The listing builds one solid part. Answer for the finished solid, in the listing's coordinates (mm). A direction names the side the tool comes from. Coordinates: 2 decimals unless noted, no trailing zeros. Loops run counter-clockwise (first coordinate to the right, second up) from the corner with the lowest first, then second, coordinate; pieces in that order, holes last. Notation, with made-up numbers: M -15,37 L 36,37 A15 cw 36,49 Z; hole C -29.5,62 d6. An arc over 180 degrees is marked long. Answer in a Markdown table with one row per item. Add a question column.
from build123d import *

# Parameters (mm, degrees)
CYLINDER_R             = 10
CYLINDER_DEPTH         = 10
CYLINDER001_R          = 2
CYLINDER001_DEPTH      = 30
CYLINDER001_ROLL_ANGLE = -90
CYLINDER003_R          = 1.5
CYLINDER003_DEPTH      = 10
CYLINDER003_ROLL_ANGLE = -90
CYLINDER002_R          = 1.5
CYLINDER002_DEPTH      = 10
CYLINDER002_ROLL_ANGLE = -90
BOX001_W               = 15
BOX001_H               = 10
BOX001_DEPTH           = 10
BOX_W                  = 35
BOX_H                  = 30
BOX_DEPTH              = 10
BOX002_W               = 68
BOX002_H               = 10
BOX002_DEPTH           = 10


with BuildPart() as cylinder:
    # Cylinder → Cylinder (new body)
    with BuildSketch(Plane.XY.offset(-5)):
        Circle(CYLINDER_R)
    extrude(amount=CYLINDER_DEPTH)


with BuildPart() as cylinder001:
    # Cylinder001 → Cylinder001 (new body)
    with BuildSketch(Plane.XY):
        Circle(CYLINDER001_R)
    extrude(amount=CYLINDER001_DEPTH)


with BuildPart() as cylinder001_1:
    # Cylinder001 roll: moved
    add(cylinder001.part.rotate(Axis((0, 0, 0), (1, 0, 0)), CYLINDER001_ROLL_ANGLE))


with BuildPart() as cylinder001_2:
    # Cylinder001 placement: moved
    add(cylinder001_1.part.moved(Location((-15, -15, 0))))


with BuildPart() as cylinder003:
    # Cylinder003 → Cylinder003 (new body)
    with BuildSketch(Plane.XY):
        Circle(CYLINDER003_R)
    extrude(amount=CYLINDER003_DEPTH)


with BuildPart() as cylinder003_1:
    # Cylinder003 roll: moved
    add(cylinder003.part.rotate(Axis((0, 0, 0), (1, 0, 0)), CYLINDER003_ROLL_ANGLE))


with BuildPart() as cylinder003_2:
    # Cylinder003 placement: moved
    add(cylinder003_1.part.moved(Location((52, 10, 0))))


with BuildPart() as cylinder002:
    # Cylinder002 → Cylinder002 (new body)
    with BuildSketch(Plane.XY):
        Circle(CYLINDER002_R)
    extrude(amount=CYLINDER002_DEPTH)


with BuildPart() as cylinder002_1:
    # Cylinder002 roll: moved
    add(cylinder002.part.rotate(Axis((0, 0, 0), (1, 0, 0)), CYLINDER002_ROLL_ANGLE))


with BuildPart() as cylinder002_2:
    # Cylinder002 placement: moved
    add(cylinder002_1.part.moved(Location((21, 10, 0))))


with BuildPart() as negative_fusion:
    # Box001 → Box001 (new body)
    with BuildSketch(Plane(origin=(-20, -5, -5), x_dir=(1, 0, 0), z_dir=(0, 0, 1))):
        with Locations((7.5, 5)):
            Rectangle(BOX001_W, BOX001_H)
    extrude(amount=BOX001_DEPTH)

    # Fusion: union Cylinder, Cylinder001, Cylinder003, Cylinder002
    add(cylinder.part)
    add(cylinder001_2.part)
    add(cylinder003_2.part)
    add(cylinder002_2.part)


with BuildPart() as cube:
    # Box → Box (new body)
    with BuildSketch(Plane(origin=(-20, -15, -5), x_dir=(1, 0, 0), z_dir=(0, 0, 1))):
        with Locations((17.5, 15)):
            Rectangle(BOX_W, BOX_H)
    extrude(amount=BOX_DEPTH)


with BuildPart() as cut:
    # Box002 → Box002 (new body)
    with BuildSketch(Plane(origin=(-10, 10, -5), x_dir=(1, 0, 0), z_dir=(0, 0, 1))):
        with Locations((34, 5)):
            Rectangle(BOX002_W, BOX002_H)
    extrude(amount=BOX002_DEPTH)

    # Fusion001: union Cube
    add(cube.part)

    # Cut: cut Negative Fusion
    add(negative_fusion.part, mode=Mode.SUBTRACT)


solid = cut.part
(1) For faces 4 (the face through (15, -3, 0)), 5 (the face through (-13, 5, 1)), 6 (the face through (-10, 17, 0)), determine the directions among +Z, -Z, +X, -X, +Y, -Y from which every point of the face is accessible in a straight line to the end or side of a thin tool.
(2) Each of these flat-tipped pins is pushed along its axis until it touches: pin 1 (3 mm diameter, centred on x = -15.5, z = -0.5, fed in from -Y); pin 2 (2.5 mm diameter, centred on x = -15, z = 0, fed in from -Y); pin 3 (4 mm diameter, centred on x = 52, z = 0, fed in from -Y); pin 4 (1 mm diameter, centred on y = -2.5, z = -2.5, fed in from +X). Where does it stop, or does it pass through?
(3) The mould has two halves that part along Y. Classify faces 1 (the face through (36, 10, 0)), 2 (the face through (-13, -5, 1)), 3 (the face through (50.8, 14.9, 0.9)): released by +Y, released by -Y, zero draft, split by the parting line, or undercut.
(4) A cutting plane is placed at C-C (x = -15). Give the vertices of the cut face in (y, z), plus the area to 3 significant figures.
(5) Straight lines are drawn through the part: line 1 (Z direction, x = -15, y = 8); line 2 (Y direction, x = -17, z = 0.5); line 3 (X direction, y = 16.5, z = 0.5). For each, find the intervals that lie inside material, in ascending order.
(6) A cutting plane is placed at B-B (z = 0). Give the vertices of the cut face in (x, y).
(7) A cutting plane is placed at A-A (x = 0). Give the vertices of the cut face in (y, z), plus the area to 3 significant figures.
(8) A cutting plane is placed at D-D (y = -12). Give the vertices of the cut face in (x, z).
Solved:
| question | item | result |
|---|---|---|
| 1 | face 4 | +Z, -Z, +X, -Y |
| 1 | face 5 | +Z, -Z, -X |
| 1 | face 6 | +Z, -Z, -X, +Y |
| 2 | pin 1 | stops at y = -15 |
| 2 | pin 2 | passes through |
| 2 | pin 3 | stops at y = 10 |
| 2 | pin 4 | stops at x = 15 |
| 3 | face 1 | released by -Y |
| 3 | face 2 | undercut |
| 3 | face 3 | zero draft |
| 4 | outline | M -15,-5 L -5,-5 L -5,-2 L -15,-2 Z; M -15,2 L -5,2 L -5,5 L -15,5 Z; M 5,-5 L 15,-5 L 15,-2 L 5,-2 Z; M 5,2 L 15,2 L 15,5 L 5,5 Z |
| 4 | area | 120 mm² |
| 5 | line 1 | z = -5 to -2, 2 to 5 |
| 5 | line 2 | y = -15 to -5, 5 to 15 |
| 5 | line 3 | x = -10 to 19.59, 22.41 to 50.59, 53.41 to 58 |
| 6 | outline | M -20,-15 L -17,-15 L -17,-5 L -20,-5 Z; M -20,5 L -17,5 L -17,15 L -20,15 Z; M -13,-15 L 15,-15 L 15,10 L 19.5,10 L 19.5,20 L -10,20 L -10,15 L -13,15 L -13,5 L -8.66,5 A10 cw long -8.66,-5 L -13,-5 Z; M 22.5,10 L 50.5,10 L 50.5,20 L 22.5,20 Z; M 53.5,10 L 58,10 L 58,20 L 53.5,20 Z |
| 7 | outline | M -15,-5 L -10,-5 L -10,5 L -15,5 Z; M 10,-5 L 20,-5 L 20,5 L 10,5 Z |
| 7 | area | 150 mm² |
| 8 | outline | M -20,-5 L 15,-5 L 15,5 L -20,5 Z; hole C -15,0 d4 |
